CAD build for the part. Positions are in the model's coordinates, mm. Coordinates: 2 decimals unless noted, no trailing zeros. Write each loop counter-clockwise with the first axis right and the second up, starting at its lowest first coordinate (ties: lowest second). Pieces come first, ordered by that corner, then holes. Notation, with made-up numbers: (17, 10) - (29, 10) arc R18 cw to (29, 34) - close; hole circle Ø10 at (56.25, -30). An arc over 180 degrees is marked (long way). Answer in a Markdown table with one row per item. Add a question column.
Q1. Band-saw the part on B-B (y = 12). List the corners of the cut face in (x, z), and give its area (3 significant figures).
Q2. Band-saw the part on C-C (x = 5.7). List the corners of the cut face in (y, z), and give its area (3 significant figures).
Q3. Band-saw the part on A-A (z = 0.5). List the corners of the cut face in (x, y).
Q4. Pin check, flat tip, straight feed: pin 1 (2 mm diameter, centred on y = 24, z = 3, fed in from -X). Stop position of the tip, or through.
Q5. Band-saw the part on D-D (y = 28.5). List the corners of the cut face in (x, z).
Q6. Drill centre lines: line 1 along Y through (x, z) = (5.7, 2.3); line 2 along X through (y, z) = (2, 1.1); line 3 along Z through (x, y) = (38.5, 13). Where is each one in solid material? Low to high. Write a range as from..to.
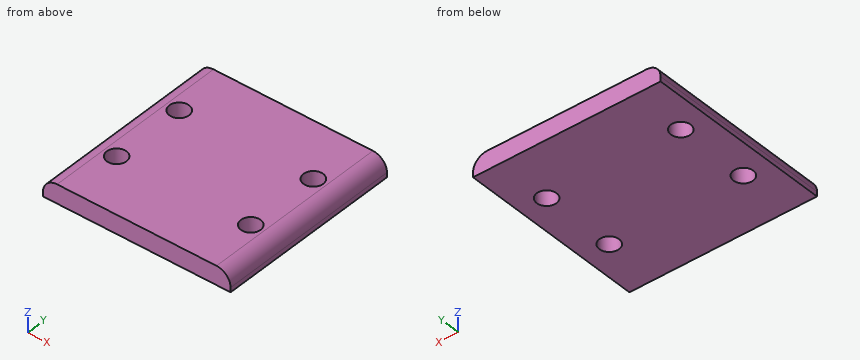
```python
from build123d import *

# Parameters (mm, degrees)
F0_W     = 40
F0_H     = 40
F1_DEPTH = 8
F2_R     = 2.1
F3_DEPTH = 25
F4_W     = 40
F4_H     = 4
F5_DEPTH = 100
F6_R     = 3


# Not quite as in the source:
# - a feature names something its author has since deleted; it is built from what else it names


with BuildPart() as f1:
    # F0 (on Top) → F1 (new body)
    with BuildSketch(Plane.XY):
        with Locations((20, 20)):
            Rectangle(F0_W, F0_H)
    extrude(amount=F1_DEPTH)

    # F2 (on face) → F3 (cut)
    with BuildSketch(Plane.XY.offset(8)):
        with Locations((5.7, 12)):
            Circle(F2_R)
        with Locations((5.7, 28)):
            Circle(F2_R)
        with Locations((34.3, 28)):
            Circle(F2_R)
        with Locations((34.3, 12)):
            Circle(F2_R)
    extrude(amount=-F3_DEPTH, mode=Mode.SUBTRACT)

    # F4 (on face) → F5 (cut)
    with BuildSketch(Plane(origin=(0, 40, 0), x_dir=(-1, 0, 0), z_dir=(0, 1, 0))):
        with Locations((-20, 6)):
            Rectangle(F4_W, F4_H)
    extrude(amount=-F5_DEPTH, mode=Mode.SUBTRACT)

    # F6
    f6_edges = [f1.edges().sort_by_distance(p)[0] for p in [
        (0, 20, 4),
        (40, 20, 4),
    ]]
    fillet(f6_edges, radius=F6_R)


solid = f1.part
```
Checked values:
| question | item | result |
|---|---|---|
| 1 | outline | (0, 0) - (3.6, 0) - (3.6, 4) - (3, 4) arc R3 ccw to (0, 1) - close; (7.8, 0) - (32.2, 0) - (32.2, 4) - (7.8, 4) - close; (36.4, 0) - (40, 0) - (40, 1) arc R3 ccw to (37, 4) - (36.4, 4) - close |
| 1 | area | 123 mm² |
| 2 | outline | (0, 0) - (9.9, 0) - (9.9, 4) - (0, 4) - close; (14.1, 0) - (25.9, 0) - (25.9, 4) - (14.1, 4) - close; (30.1, 0) - (40, 0) - (40, 4) - (30.1, 4) - close |
| 2 | area | 126 mm² |
| 3 | outline | (0, 0) - (40, 0) - (40, 40) - (0, 40) - close; hole circle Ø4.2 at (5.7, 12); hole circle Ø4.2 at (5.7, 28); hole circle Ø4.2 at (34.3, 12); hole circle Ø4.2 at (34.3, 28) |
| 4 | pin 1 | stops at x = 0.17 |
| 5 | outline | (0, 0) - (3.66, 0) - (3.66, 4) - (3, 4) arc R3 ccw to (0, 1) - close; (7.74, 0) - (32.26, 0) - (32.26, 4) - (7.74, 4) - close; (36.34, 0) - (40, 0) - (40, 1) arc R3 ccw to (37, 4) - (36.34, 4) - close |
| 6 | line 1 | y = 0..9.9, 14.1..25.9, 30.1..40 |
| 6 | line 2 | x = 0..40 |
| 6 | line 3 | z = 0..3.6 |
